Check sheet for the modelled part. Datum: model origin and axes. Units: mm. Face numbers are marked on the shaded views. Round coordinates to 2 decimals unless told otherwise and drop trailing zeros. Order: outer loops, then holes, each group sorted by start corner. A loop starts at its lowest first (then second) coordinate and runs counter-clockwise, first axis right, second up.
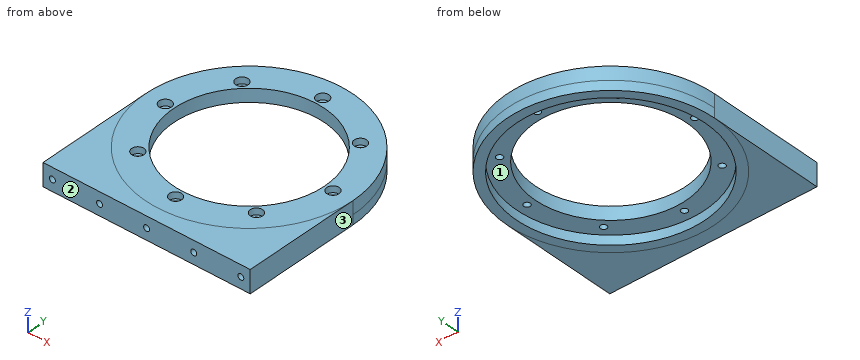
from build123d import *

# Parameters (mm, degrees)
SKETCH1_R                                           = 55
SKETCH1_R_2                                         = 40
BOSS_EXTRUDE1_DEPTH                                 = 7
CBORE_FOR_M3_HEX_SOCKET_HEAD_CAP_SCREW1_D           = 3.4
CBORE_FOR_M3_HEX_SOCKET_HEAD_CAP_SCREW1_CBORE_D     = 6.5
CBORE_FOR_M3_HEX_SOCKET_HEAD_CAP_SCREW1_CBORE_DEPTH = 3.4
BOSS_EXTRUDE3_START                                 = 5
SKETCH4_R                                           = 55
SKETCH4_R_2                                         = 50
BOSS_EXTRUDE3_DEPTH                                 = 5
BOSS_EXTRUDE4_START                                 = -12
BOSS_EXTRUDE4_DEPTH                                 = 12
TAP_DRILL_FOR_M3_HELICOIL1_D                        = 3.15
TAP_DRILL_FOR_M3_HELICOIL1_DEPTH                    = 10
TAP_DRILL_FOR_M3_HELICOIL1_TIP                      = 0.946355475


with BuildPart() as part:
    # Sketch1 → Boss-Extrude1 (new body)
    with BuildSketch(Plane.XY):
        Circle(SKETCH1_R)
        Circle(SKETCH1_R_2, mode=Mode.SUBTRACT)
    extrude(amount=BOSS_EXTRUDE1_DEPTH)

    # CBORE for M3 Hex Socket Head Cap Screw1 (through all)
    with Locations(Plane.XY.offset(7)):
        with Locations((-31.466251763, 31.466251763), (0, 44.5), (31.466251763, 31.466251763), (44.5, 0), (31.466251763, -31.466251763), (0, -44.5), (-31.466251763, -31.466251763), (-44.5, 0)):
            CounterBoreHole(CBORE_FOR_M3_HEX_SOCKET_HEAD_CAP_SCREW1_D / 2, CBORE_FOR_M3_HEX_SOCKET_HEAD_CAP_SCREW1_CBORE_D / 2, CBORE_FOR_M3_HEX_SOCKET_HEAD_CAP_SCREW1_CBORE_DEPTH)

    # Sketch4 → Boss-Extrude3 (add)
    with BuildSketch(Plane(origin=(0, 0, 0), x_dir=(-1, 0, 0), z_dir=(0, 0, -1)).offset(BOSS_EXTRUDE3_START)):
        Circle(SKETCH4_R)
        Circle(SKETCH4_R_2, mode=Mode.SUBTRACT)
    extrude(amount=-BOSS_EXTRUDE3_DEPTH)

    # Sketch5 → Boss-Extrude4 (add)
    with BuildSketch(Plane.XY.offset(7).offset(BOSS_EXTRUDE4_START)):
        with BuildLine():
            Line((-55, 0), (-55, -62))
            Line((-55, -62), (55, -62))
            Line((55, -62), (55, 0))
            ThreePointArc((55, 0), (0, -55), (-55, 0))
        make_face()
    extrude(amount=BOSS_EXTRUDE4_DEPTH)

    # Tap Drill for M3 Helicoil1
    with Locations(Plane(origin=(0, -62, 0), x_dir=(-1, 0, 0), z_dir=(0, -1, 0))):
        with Locations((-50, -1), (0, -1), (25, -1), (50, -1), (-25, -1)):
            Hole(TAP_DRILL_FOR_M3_HELICOIL1_D / 2, depth=TAP_DRILL_FOR_M3_HELICOIL1_DEPTH)
            with Locations((0, 0, -(TAP_DRILL_FOR_M3_HELICOIL1_DEPTH + TAP_DRILL_FOR_M3_HELICOIL1_TIP / 2))):  # 118° drill point
                Cone(0, TAP_DRILL_FOR_M3_HELICOIL1_D / 2, TAP_DRILL_FOR_M3_HELICOIL1_TIP, mode=Mode.SUBTRACT)


solid = part.part
1) Sectioned sample at B-B on x = 37.5. Record the cut outline in (y, z).
2) Sectioned sample at A-A on y = 25. Record the cut outline in (x, z).
3) Draft check along X on the marked faces 1, 2 and 3. Enter one of: pulls with the +X half, pulls with the -X half, needs draft (parallel to the pull), parting line crosses it, or undercut.
4) Gauge pin test, flat ends, axial feed: pin 1 (7.5 mm diameter, centred on x = 0, y = 44.5, fed in from -Z); pin 2 (10.5 mm diameter, centred on x = -31.47, y = 31.47, fed in from +Z); pin 3 (3 mm diameter, centred on x = -44.5, y = 0, fed in from +Z); pin 4 (3.5 mm diameter, centred on x = 32.5, y = 30.5, fed in from +Z). Record the tip position at first contact, or that the pin passes through.
5) Scan lines: line 1 (Z direction, x = -25, y = -54.5) (3 decimals); line 2 (X direction, y = 32, z = 4.75); line 3 (Y direction, x = 0, z = 0.75). Record each from-to range of solid material in increasing order.
6) Sectioned sample at C-C on y = -44.5. Record the cut outline in (x, z), and give its area (3 significant figures).
Values found:
1. outline: (-62, -5) - (-33.07, -5) - (-33.07, 0) - (-13.92, 0) - (-13.92, 7) - (-62, 7) - close; (13.92, 0) - (33.07, 0) - (33.07, -5) - (40.23, -5) - (40.23, 7) - (13.92, 7) - close
2. outline: (-48.99, -5) - (-43.3, -5) - (-43.3, 0) - (-31.22, 0) - (-31.22, 7) - (-48.99, 7) - close; (31.22, 0) - (43.3, 0) - (43.3, -5) - (48.99, -5) - (48.99, 7) - (31.22, 7) - close
3. face 1: undercut
3. face 2: needs draft
3. face 3: pulls with the +X half
4. pin 1: stops at z = 0
4. pin 2: stops at z = 7
4. pin 3: passes through
4. pin 4: stops at z = 3.6
5. line 1: z = -5 to -0.575, 2.575 to 7
5. line 2: x = -44.73 to -34.67, -28.26 to -24, 24 to 28.26, 34.67 to 44.73
5. line 3: y = -51.2 to -46.2, -42.8 to -40, 40 to 42.8, 46.2 to 55
6. outline: (-55, -5) - (-22.8, -5) - (-22.8, 0) - (-1.7, 0) - (-1.7, 3.6) - (-3.25, 3.6) - (-3.25, 7) - (-55, 7) - close; (1.7, 0) - (22.8, 0) - (22.8, -5) - (55, -5) - (55, 7) - (3.25, 7) - (3.25, 3.6) - (1.7, 3.6) - close
6. area: 1,060 mm2
